Solid Edge part; units mm, degrees
sketch "Sketch1" plane through (0, 0, 0) normal (0, -1, 0) x (1, 0, 0)
  circle A0 centre (0, 0) radius 7.5
extrude "Protrusion1" add sketch "Sketch1" against normal blind 82
sketch "Sketch2" plane through (0, 0, 0) normal (0, -1, 0) x (1, 0, 0)
  line L0 (-6, -6) -> (6, -6)
  line L1 (6, -6) -> (6, 6)
  line L2 (6, 6) -> (-6, 6)
  line L3 (-6, 6) -> (-6, -6)
  circle A0 centre (0, 0) radius 11.1148
  dimension "D1" = 6
  dimension "D2" = 6
extrude "VaciadoExtruido_1" cut sketch "Sketch2" against normal blind 14.5
sketch "Sketch3" plane through (0, 82, 0) normal (0, 1, 0) x (-1, 0, 0)
  line L0 (-6, 6) -> (6, 6)
  line L1 (6, 6) -> (6, -6)
  line L2 (6, -6) -> (-6, -6)
  line L3 (-6, -6) -> (-6, 6)
  circle A0 centre (0, 0) radius 11.8387
  dimension "D1" = 6
  dimension "D2" = 6
extrude "VaciadoExtruido_2" cut sketch "Sketch3" against normal blind 8
hole "Agujero_1" at (0, 0, 0) direction (0, 1, 0) diameter 4.917 depth 20 tip angle 118 thread major 6 thread length 15
hole "Agujero_2" at (0, 82, 0) direction (0, -1, 0) diameter 4.917 depth 20 tip angle 118 thread major 6 thread length 15
properties part number "1976-1300-007"
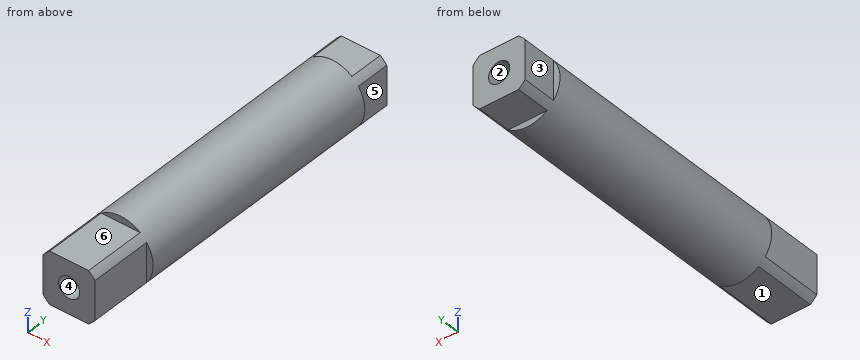
Can you work these out from the model? Positions are in its coordinate system, mm. Face numbers are marked on the shaded views. A direction names the side the tool comes from. Coordinates: 2 decimals unless noted, no trailing zeros. Write each loop counter-clockwise with the first axis right and the second up, starting at its lowest first coordinate (ties: lowest second). Pieces come first, ordered by that corner, then holes. Notation, with made-up numbers: (57, 36.25) - (66, 36.25) arc R38 cw to (66, 74.25) - close; hole circle Ø5 at (28, 75.5). An arc over 180 degrees is marked (long way). Return JSON: item names as keys, results as strings.
Q1. Please list where these lines run through material, in increasing order: L1, parallel to X at y = 11.5, z = 0; L2, parallel to Y at x = 3.5, z = 6.5. Write a range as from..to.
Computed values:
{"L1": "x = -6..-2.46, 2.46..6", "L2": "y = 14.5..74"}
Q2. If we section it at A-A (y = 34.5): Please give me the cut outline in (x, z), then the cut area to 3 significant figures.
Computed values:
{"outline": "circle Ø15 at (0, 0)", "area": "177 mm2"}
Q3. I'm going to push flat-ended pins straight in: pin 1 Ø4.5 at (x, z) = (0, 0) entering from +Y; pin 2 Ø2 at (y, z) = (39.5, -5) entering from +X; pin 3 Ø2.5 at (x, y) = (1, 76) entering from +Z. Where does each tip first touch, or does it pass through?
Computed values:
{"pin 1": "stops at y = 61.87", "pin 2": "stops at x = 6.34", "pin 3": "stops at z = 6"}
Q4. If we section it at B-B (x = 6.75): Please give me the cut outline in (y, z), then the cut area to 3 significant figures.
Computed values:
{"outline": "(14.5, -3.27) - (74, -3.27) - (74, 3.27) - (14.5, 3.27) - close", "area": "389 mm2"}
Q5. Thinking about a two-plate mould opening in Z: for the marked faces 1, 2 and 3, which applies, +Z half, -Z half, draft (parallel to the pull), parting line (faces both ways), or undercut?
Computed values:
{"face 1": "-Z half", "face 2": "undercut", "face 3": "draft"}
Q6. On a 3-axis mill with a long thin cutter (end or side, diameter ignored), from which of +Z, -Z, +X, -X, +Y, -Y can I reach the whole of each face in a straight line? I mean the marked faces 4, 5 and 6. Say none if no direction works.
Computed values:
{"face 4": "-Y", "face 5": "+Z, -Z, +X, +Y", "face 6": "+Z, +X, -X, -Y"}
